Print and shaded views of the part. All mm, measured from the part's lowest x, y and z. Coordinates: 2 decimals unless noted, no trailing zeros. Loops run counter-clockwise (first coordinate to the right, second up) from the corner with the lowest first, then second, coordinate; pieces in that order, holes last. Notation, with made-up numbers: M -10.5,47 L 28.5,47 A19 cw 28.5,52 Z; hole C -10.75,-20.5 d6. An arc over 180 degrees is marked long. Use a Markdown table: item, result. Add a question column.
1) Band-saw the part on A-A (y = 11). List the corners of the cut face in (x, z), plus the area to 3 significant figures.
2) Wall check: probe 1 along Y at (x, z) = (6, 52.5); probe 2 along X at (y, z) = (6.5, 89); probe 3 along X at (y, z) = (7.5, 83.5) (3 decimals). Give the ranges that are in metal, low to high. Write a range as from..to.
3) Pin check, flat tips, straight feed: pin 1 Ø2 at (x, z) = (3, 25) entering from +Y; pin 2 Ø1.5 at (x, z) = (2.5, 81.5) entering from -Y. Stop position of each tip, or through.
4) Band-saw the part on B-B (z = 27.5). List the corners of the cut face in (x, y).
5) Band-saw the part on C-C (x = 11.75). List the corners of the cut face in (y, z).
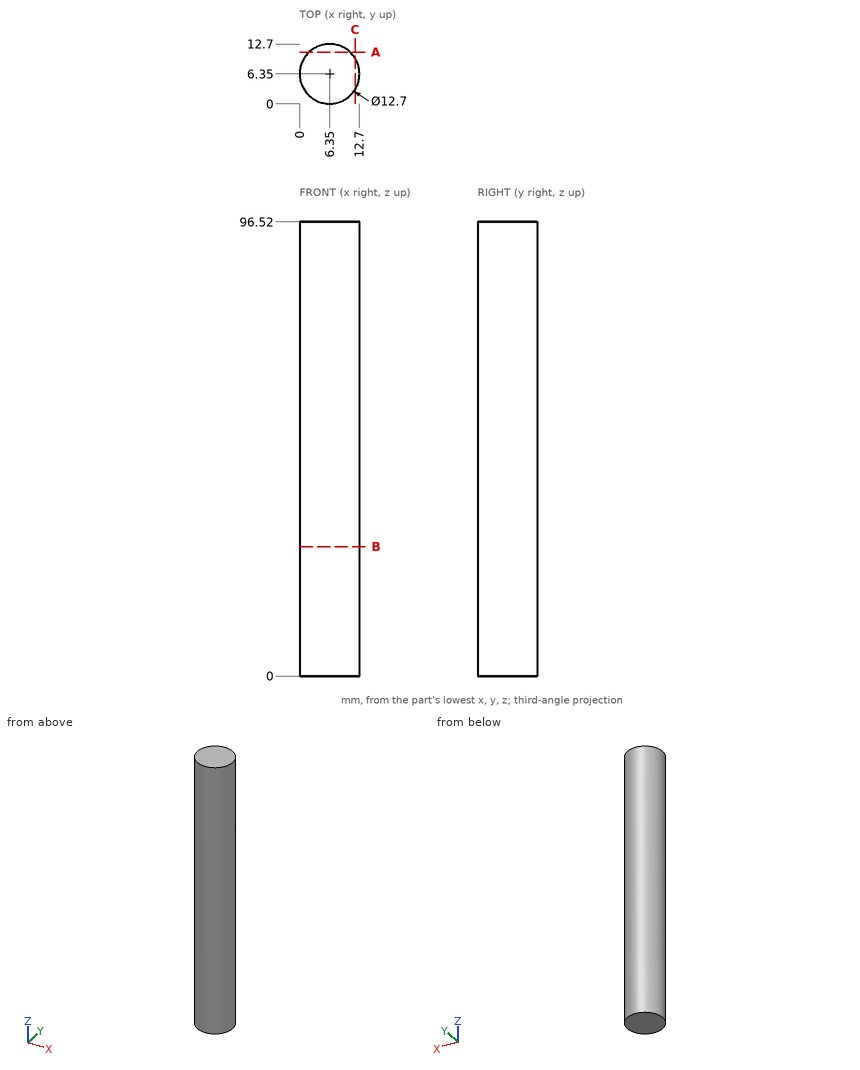
Entries:
| question | item | result |
|---|---|---|
| 1 | outline | M 2.03,0 L 10.67,0 L 10.67,96.52 L 2.03,96.52 Z |
| 1 | area | 835 mm2 |
| 2 | probe 1 | 0.01..12.69 |
| 2 | probe 2 | 0..12.7 |
| 2 | probe 3 | 0.105..12.595 |
| 3 | pin 1 | y = 12.25 |
| 3 | pin 2 | y = 0.81 |
| 4 | outline | C 6.35,6.35 d12.7 |
| 5 | outline | M 3.01,0 L 9.69,0 L 9.69,96.52 L 3.01,96.52 Z |
